Build history of the part. All positions in model axes, mm. Face numbers are marked on the shaded views. A direction names the side the tool comes from. Give positions to 0.01 mm unless a question says otherwise; leave off trailing zeros. Loops run counter-clockwise (first coordinate to the right, second up) from the corner with the lowest first, then second, coordinate; pieces in that order, holes last. Notation, with made-up numbers: (9, -15.5) -> (27, -15.5) arc R31 ccw to (27, 21.5) -> close; hole circle Ø8 at (75.5, -6.75). An arc over 180 degrees is marked (long way). Answer in a Markdown table with one row per item. Add a question column.
from build123d import *

# Parameters (mm, degrees)
F0_W      = 41.100144
F0_H      = 24.865199
F1_DEPTH  = 26.924
F3_DEPTH  = 33.02
F5_DEPTH  = 9.906
F6_R      = 5.08
F7_R      = 2.565784
F7_R_2    = 2.684089
F7_R_3    = 0.988896
F8_DEPTH  = 25.4
F10_R     = 3.124408
F11_DEPTH = 20.574
F12_SIZE  = 1.27


with BuildPart() as f1:
    # F0 (on Top) → F1 (new body)
    with BuildSketch(Plane.XY):
        with Locations((20.550072, 12.4326)):
            Rectangle(F0_W, F0_H)
    extrude(amount=F1_DEPTH)

    # F2 (on Front) → F3 (cut)
    with BuildSketch(Plane.XZ):
        with BuildLine():
            Line((11.39266, 0), (25.158048, 0))
            ThreePointArc((25.158048, 0), (18.275354, 6.882694), (11.39266, 0))
        make_face()
        with BuildLine():
            ThreePointArc((8.551842, 5.420331), (18.231203, 11.132148), (27.955566, 5.497288))
            Line((27.955566, 5.497288), (35.856735, 5.497288))
            Line((35.856735, 5.497288), (35.856735, 20.804519))
            Line((35.856735, 20.804519), (43.18231, 20.804519))
            Line((43.18231, 20.804519), (42.240448, 32.735568))
            Line((42.240448, 32.735568), (-4.643232, 32.735568))
            Line((-4.643232, 32.735568), (0, 5.420331))
            Line((0, 5.420331), (8.551842, 5.420331))
        make_face()
    extrude(amount=-F3_DEPTH, mode=Mode.SUBTRACT)

    # F4 (on face) → F5 (cut)
    with BuildSketch(Plane.YZ.offset(41.100144)):
        with BuildLine():
            Line((9.614374, 20.804519), (9.614374, 12.291135))
            ThreePointArc((9.614374, 12.291135), (12.13957, 9.414848), (14.903929, 12.062103))
            Line((14.903929, 12.062103), (15.042416, 20.804519))
            Line((15.042416, 20.804519), (9.614374, 20.804519))
        make_face()
    extrude(amount=-F5_DEPTH, mode=Mode.SUBTRACT)

    # F6
    f6_edges = [f1.edges().sort_by_distance(p)[0] for p in [
        (38.47844, 0, 20.804519),
        (38.47844, 24.865199, 20.804519),
        (0, 24.865199, 2.710165),
        (0, 0, 2.710165),
    ]]
    fillet(f6_edges, radius=F6_R)

    # F7 (on face) → F8 (cut)
    with BuildSketch(Plane(origin=(0, 0, 0), x_dir=(1, 0, 0), z_dir=(0, 0, -1))):
        with Locations((5.08, -5.08)):
            Circle(F7_R)
        with Locations((5.08, -19.785199)):
            Circle(F7_R_2)
        with Locations((17.942235, -12.616471)):
            Circle(F7_R_3)
    extrude(amount=-F8_DEPTH, mode=Mode.SUBTRACT)

    # F10 (on offset) → F11 (cut)
    with BuildSketch(Plane.XY.offset(29.718)):
        with Locations((17.889135, 12.645945)):
            Circle(F10_R)
    extrude(amount=-F11_DEPTH, mode=Mode.SUBTRACT)

    # F12
    f12_edges = [f1.edges().sort_by_distance(p)[0] for p in [
        (14.764727, 12.645945, 9.144),
    ]]
    chamfer(f12_edges, length=F12_SIZE)


solid = f1.part
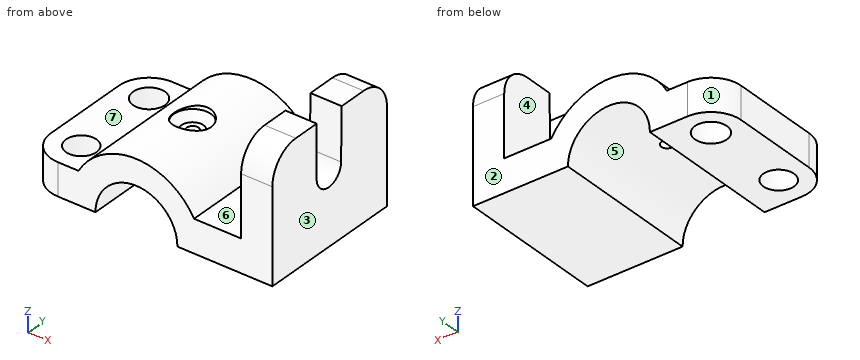
(1) Saw through at A-A, the plane z = 5. List the corners of the cut face in (x, y), then the cut area to 3 significant figures.
(2) Saw through at B-B, the plane y = 5.75. List the corners of the cut face in (x, z).
(3) Flat gauge pins, fed straight in: pin 1 Ø5 at (x, y) = (7.5, 19) entering from -Z; pin 2 Ø1.6 at (x, z) = (39.5, 18) entering from +Y; pin 3 Ø3 at (x, y) = (17, 13) entering from +Z; pin 4 Ø5 at (x, y) = (17.89, 12.65) entering from +Z. Where does each tip first touch, or does it go through?
(4) Wall check: line 1 along Y through (x, z) = (5.08, 1.9); line 2 along X through (y, z) = (21.25, 5.75); line 3 along X through (y, z) = (16.75, 6.25). Give the ranges that are in metal, low to high. Write a range as from..to.
(5) Two-plate mould, pull along X, no slides. Class the marked faces 1, 2, 3 and 4: released by +X, released by -X, zero draft, split by the parting line, or undercut.
(6) Saw through at D-D, the plane z = 13.5. List the corners of the cut face in (x, y).
(7) 3-axis set-ups, long thin cutter, end or side, ignore diameter. For the marked faces 5, 6 and 7: which of +Z, -Z, +X, -X, +Y, -Y reach the whole face in a straight line?
(8) Saw through at C-C, the plane x = 7. List the corners of the cut face in (y, z), then the cut area to 3 significant figures.
Worked answers:
| question | item | result |
|---|---|---|
| 1 | outline | (0, 5.08) arc R5.08 ccw to (5.08, 0) -> (13.55, 0) -> (13.55, 24.87) -> (5.08, 24.87) arc R5.08 ccw to (0, 19.79) -> close; (23.01, 0) -> (41.1, 0) -> (41.1, 24.87) -> (23.01, 24.87) -> close; hole circle Ø5.37 at (5.08, 19.79); hole circle Ø5.13 at (5.08, 5.08) |
| 1 | area | 732 mm^2 |
| 2 | outline | (0, 0) -> (2.6, 0) -> (2.6, 5.42) -> (0, 5.42) -> close; (7.56, 0) -> (11.39, 0) arc R6.88 cw to (25.16, 0) -> (41.1, 0) -> (41.1, 20.8) -> (35.86, 20.8) -> (35.86, 5.5) -> (27.96, 5.5) arc R11.13 ccw to (8.55, 5.42) -> (7.56, 5.42) -> close |
| 3 | pin 1 | z = 0 |
| 3 | pin 2 | y = 24.65 |
| 3 | pin 3 | z = 9.75 |
| 3 | pin 4 | z = 9.79 |
| 4 | line 1 | 0..2.51, 7.65..17.1, 22.47..24.87 |
| 4 | line 2 | 8.74..14.49, 22.06..27.81, 35.86..41.1 |
| 4 | line 3 | 9.06..15.39, 21.16..27.49, 35.86..41.1 |
| 5 | face 1 | released by -X |
| 5 | face 2 | zero draft |
| 5 | face 3 | released by +X |
| 5 | face 4 | undercut |
| 6 | outline | (35.86, 0) -> (41.1, 0) -> (41.1, 9.61) -> (35.86, 9.61) -> close; (35.86, 14.93) -> (41.1, 14.93) -> (41.1, 24.87) -> (35.86, 24.87) -> close |
| 7 | face 5 | -Z, +Y, -Y |
| 7 | face 6 | +Z, +Y, -Y |
| 7 | face 7 | +Z, -X, +Y, -Y |
| 8 | outline | (0, 0) -> (3.38, 0) -> (3.38, 5.42) -> (0, 5.42) -> close; (6.78, 0) -> (17.91, 0) -> (17.91, 5.42) -> (6.78, 5.42) -> close; (21.66, 0) -> (24.87, 0) -> (24.87, 5.42) -> (21.66, 5.42) -> close |
| 8 | area | 96.0 mm^2 |
